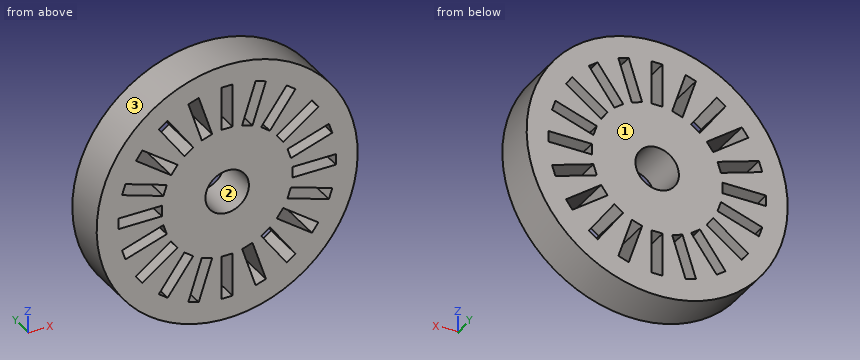
```python
from build123d import *

# Parameters (mm, degrees)
SKETCH1_R           = 12
SKETCH1_R_2         = 2
BOSS_EXTRUDE1_DEPTH = 4


with BuildPart() as part:
    # Sketch1 → Boss-Extrude1 (new body)
    with BuildSketch(Plane(origin=(0, 0, 0), x_dir=(1, 0, 0), z_dir=(0, 1, 0))):
        with Locations(Location((0, 0, 0), (0, 0, 270))):
            Circle(SKETCH1_R)
        Polygon((-5.473344026, -8.38406257), (-5.877852523, -8.090169944), (-6.28236102, -7.796277318), (-3.931220011, -4.56020934), (-3.122203017, -5.147994592), align=None, mode=Mode.SUBTRACT)
        Polygon((-2.614641686, -9.66507366), (-3.090169944, -9.510565163), (-3.565698202, -9.356056666), (-2.329630224, -5.551830601), (-1.378573708, -5.860847595), align=None, mode=Mode.SUBTRACT)
        Polygon((-7.796277318, -6.28236102), (-8.090169944, -5.877852523), (-8.38406257, -5.473344026), (-5.147994592, -3.122203017), (-4.56020934, -3.931220011), align=None, mode=Mode.SUBTRACT)
        Polygon((-9.356056666, -3.565698202), (-9.510565163, -3.090169944), (-9.66507366, -2.614641686), (-5.860847595, -1.378573708), (-5.551830601, -2.329630224), align=None, mode=Mode.SUBTRACT)
        Polygon((0.5, -10), (0, -10), (-0.5, -10), (-0.5, -6), (0.5, -6), align=None, mode=Mode.SUBTRACT)
        Polygon((3.565698202, -9.356056666), (3.090169944, -9.510565163), (2.614641686, -9.66507366), (1.378573708, -5.860847595), (2.329630224, -5.551830601), align=None, mode=Mode.SUBTRACT)
        Polygon((6.28236102, -7.796277318), (5.877852523, -8.090169944), (5.473344026, -8.38406257), (3.122203017, -5.147994592), (3.931220011, -4.56020934), align=None, mode=Mode.SUBTRACT)
        Polygon((8.38406257, -5.473344026), (8.090169944, -5.877852523), (7.796277318, -6.28236102), (4.56020934, -3.931220011), (5.147994592, -3.122203017), align=None, mode=Mode.SUBTRACT)
        Polygon((9.66507366, -2.614641686), (9.510565163, -3.090169944), (9.356056666, -3.565698202), (5.551830601, -2.329630224), (5.860847595, -1.378573708), align=None, mode=Mode.SUBTRACT)
        Polygon((10, 0.5), (10, 0), (10, -0.5), (6, -0.5), (6, 0.5), align=None, mode=Mode.SUBTRACT)
        Polygon((-10, -0.5), (-10, 0), (-10, 0.5), (-6, 0.5), (-6, -0.5), align=None, mode=Mode.SUBTRACT)
        Polygon((-9.66507366, 2.614641686), (-9.510565163, 3.090169944), (-9.356056666, 3.565698202), (-5.551830601, 2.329630224), (-5.860847595, 1.378573708), align=None, mode=Mode.SUBTRACT)
        Polygon((-8.38406257, 5.473344026), (-8.090169944, 5.877852523), (-7.796277318, 6.28236102), (-4.56020934, 3.931220011), (-5.147994592, 3.122203017), align=None, mode=Mode.SUBTRACT)
        Polygon((-6.28236102, 7.796277318), (-5.877852523, 8.090169944), (-5.473344026, 8.38406257), (-3.122203017, 5.147994592), (-3.931220011, 4.56020934), align=None, mode=Mode.SUBTRACT)
        Polygon((-3.565698202, 9.356056666), (-3.090169944, 9.510565163), (-2.614641686, 9.66507366), (-1.378573708, 5.860847595), (-2.329630224, 5.551830601), align=None, mode=Mode.SUBTRACT)
        with Locations(Location((0, 0, 0), (0, 0, 270))):
            Circle(SKETCH1_R_2, mode=Mode.SUBTRACT)
        Polygon((9.356056666, 3.565698202), (9.510565163, 3.090169944), (9.66507366, 2.614641686), (5.860847595, 1.378573708), (5.551830601, 2.329630224), align=None, mode=Mode.SUBTRACT)
        Polygon((7.796277318, 6.28236102), (8.090169944, 5.877852523), (8.38406257, 5.473344026), (5.147994592, 3.122203017), (4.56020934, 3.931220011), align=None, mode=Mode.SUBTRACT)
        Polygon((-0.5, 10), (0, 10), (0.5, 10), (0.5, 6), (-0.5, 6), align=None, mode=Mode.SUBTRACT)
        Polygon((2.614641686, 9.66507366), (3.090169944, 9.510565163), (3.565698202, 9.356056666), (2.329630224, 5.551830601), (1.378573708, 5.860847595), align=None, mode=Mode.SUBTRACT)
        Polygon((5.473344026, 8.38406257), (5.877852523, 8.090169944), (6.28236102, 7.796277318), (3.931220011, 4.56020934), (3.122203017, 5.147994592), align=None, mode=Mode.SUBTRACT)
    extrude(amount=BOSS_EXTRUDE1_DEPTH)


solid = part.part
```
Read the model definition and answer for the solid it produces. Units are mm, in the model's axes. Face numbers are marked on the shaded views. Give positions to 0.01 mm unless a question says otherwise; leave off trailing zeros. Loops run counter-clockwise (first coordinate to the right, second up) from the corner with the lowest first, then second, coordinate; pieces in that order, holes last.
Item 1: The part is cut by section D-D (y = 1.75). Give the number of separate pieces and of enclosed holes in the cut face, and give its area (3 significant figures).
Item 2: The part is cut by section B-B (x = 0). Write down the section's boundary in (y, z).
Item 3: Find the intervals of material crossed by line 1 along X through (y, z) = (1.85, 0); line 2 along X through (y, z) = (1.15, 5.5); line 3 along Z through (x, y) = (7.75, 2.8), in increasing order.
Item 4: The mould has two halves that part along X. Classify the marked faces 1, 2 and 3: released by +X, released by -X, zero draft, split by the parting line, or undercut.
Item 5: Each of these flat-tipped pins is pushed along its axis until it touches: pin 1 Ø2 at (y, z) = (3, 8.5) entering from -X; pin 2 Ø2 at (y, z) = (2.5, -9) entering from +X; pin 3 Ø2 at (y, z) = (3.5, -5.5) entering from +X. Where does it stop, or does it pass through?
Item 6: The part is cut by section A-A (z = 0). Write down the section's boundary in (x, y), and give its area (3 significant figures).
Item 7: The part is cut by section C-C (z = -4.25). Write down the section's boundary in (x, y), and give its area (3 significant figures).
Taken from the geometry:
1. separate pieces: 1
1. enclosed holes: 21
1. area: 360 mm2
2. outline: (0, -12) - (4, -12) - (4, -10) - (0, -10) - close; (0, -6) - (4, -6) - (4, -2) - (0, -2) - close; (0, 2) - (4, 2) - (4, 6) - (0, 6) - close; (0, 10) - (4, 10) - (4, 12) - (0, 12) - close
3. line 1: x = -12 to -10, -6 to -2, 2 to 6, 10 to 12
3. line 2: x = -10.67 to -8.36, -6.72 to -4.61, -3.38 to 3.38, 4.61 to 6.72, 8.36 to 10.67
3. line 3: z = -9.16 to -6.25, -5.01 to -3.04, -1.99 to -0.5, 0.5 to 1.99, 3.04 to 5.01, 6.25 to 9.16
4. face 1: zero draft
4. face 2: undercut
4. face 3: split by the parting line
5. pin 1: stops at x = -9.37
5. pin 2: stops at x = 8.94
5. pin 3: stops at x = 11.12
6. outline: (-12, 0) - (-10, 0) - (-10, 4) - (-12, 4) - close; (-6, 0) - (-2, 0) - (-2, 4) - (-6, 4) - close; (2, 0) - (6, 0) - (6, 4) - (2, 4) - close; (10, 0) - (12, 0) - (12, 4) - (10, 4) - close
6. area: 48.0 mm2
7. outline: (-11.22, 0) - (-6.7, 0) - (-6.7, 4) - (-11.22, 4) - close; (-5, 0) - (5, 0) - (5, 4) - (-5, 4) - close; (6.7, 0) - (11.22, 0) - (11.22, 4) - (6.7, 4) - close
7. area: 76.2 mm2
